Geometry check sheet. Reference: the model listing, model coordinates, mm. Face numbers are marked on the shaded views. Round coordinates to 2 decimals unless told otherwise and drop trailing zeros. Order: outer loops, then holes, each group sorted by start corner. A loop starts at its lowest first (then second) coordinate and runs counter-clockwise, first axis right, second up. Notation, with made-up numbers: M -17.75,-27.75 L -4.75,-27.75 A21 ccw -4.75,-0.75 Z; hole C 48.5,38 d10. An arc over 180 degrees is marked long. Answer as a JSON object with one key per item and string values. Group by question number.
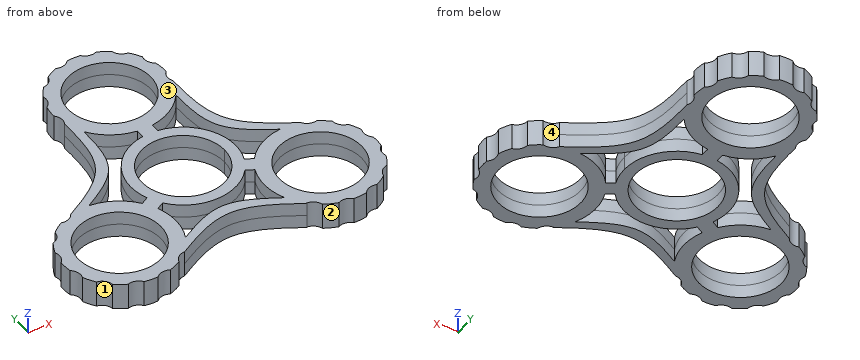
```python
from build123d import *

# Parameters (mm, degrees)
F0_R     = 11
F1_DEPTH = 3.5


with BuildPart() as f1:
    # F0 (on Top) → F1 (new body, symmetric)
    with BuildSketch(Plane.XY):
        with BuildLine():
            ThreePointArc((-12.2872806643, 22.3963534547), (-7.7936356612, 18.1836337763), (-1.9858156028, 16.1320298497))
            ThreePointArc((-1.9858156028, 16.1320298497), (0, 16), (1.9858156028, 16.1320298497))
            ThreePointArc((1.9858156028, 16.1320298497), (7.7936356612, 18.1836337763), (12.2872806643, 22.3963534547))
            ThreePointArc((12.2872806643, 22.3963534547), (13.5946168055, 24.6607260739), (14.4888873943, 27.1177143235))
            ThreePointArc((14.4888873943, 27.1177143235), (14.1339131395, 28.0975622646), (14.1302209633, 29.1397211187))
            ThreePointArc((14.1302209633, 29.1397211187), (14.4333080068, 30.0392190625), (14.9986885379, 30.8016514607))
            ThreePointArc((14.9986885379, 30.8016514607), (14.9056831484, 32.6794671415), (14.5785033995, 34.5308977089))
            ThreePointArc((14.5785033995, 34.5308977089), (13.3272676617, 36.0455189605), (13.2617309026, 38.0090294241))
            ThreePointArc((13.2617309026, 38.0090294241), (12.3374426401, 39.5315595938), (11.2392015408, 40.9337983031))
            ThreePointArc((11.2392015408, 40.9337983031), (9.4252297695, 41.6882350601), (8.449800871, 43.3935816147))
            ThreePointArc((8.449800871, 43.3935816147), (6.9211928061, 44.3077830663), (5.2949987863, 45.0343502825))
            ThreePointArc((5.2949987863, 45.0343502825), (3.3387137913, 44.8537473316), (1.6794671415, 45.9056831484))
            ThreePointArc((1.6794671415, 45.9056831484), (-0.0991764374, 45.9996721309), (-1.8764216697, 45.8821719422))
            ThreePointArc((-1.8764216697, 45.8821719422), (-3.5216132547, 44.8083874871), (-5.4801153655, 44.9631062297))
            ThreePointArc((-5.4801153655, 44.9631062297), (-7.0965596362, 44.2150989906), (-8.612945352, 43.2807643232))
            ThreePointArc((-8.612945352, 43.2807643232), (-9.5657387682, 41.562668542), (-11.3695758472, 40.7843111692))
            ThreePointArc((-11.3695758472, 40.7843111692), (-12.4491787931, 39.3676727576), (-13.3532534686, 37.8330536221))
            ThreePointArc((-13.3532534686, 37.8330536221), (-13.3928205357, 35.8688482218), (-14.6239186827, 34.3378140093))
            ThreePointArc((-14.6239186827, 34.3378140093), (-14.9164615787, 32.580877595), (-14.9986885379, 30.8016514607))
            ThreePointArc((-14.9986885379, 30.8016514607), (-14.1158588279, 29.0465787811), (-14.4888873943, 27.1177143235))
            ThreePointArc((-14.4888873943, 27.1177143235), (-13.5946168055, 24.6607260739), (-12.2872806643, 22.3963534547))
        make_face()
        with Locations((0, 31)):
            Circle(F0_R, mode=Mode.SUBTRACT)
        with BuildLine():
            Line((-1.9858156028, 16.1320298497), (-1.9858156028, 13.8584463917))
            ThreePointArc((-1.9858156028, 13.8584463917), (0, 14), (1.9858156028, 13.8584463917))
            Line((1.9858156028, 13.8584463917), (1.9858156028, 16.1320298497))
            ThreePointArc((1.9858156028, 16.1320298497), (0, 16), (-1.9858156028, 16.1320298497))
        make_face()
        with BuildLine():
            ThreePointArc((12.9946744336, -5.2094564366), (12.124355653, -7), (11.0088588308, -8.6489899551))
            Line((11.0088588308, -8.6489899551), (12.977839863, -9.7857816841))
            ThreePointArc((12.977839863, -9.7857816841), (13.8564064606, -8), (14.9636554658, -6.3462481655))
            Line((14.9636554658, -6.3462481655), (12.9946744336, -5.2094564366))
        make_face()
        with BuildLine():
            ThreePointArc((-11.0088588308, -8.6489899551), (-12.124355653, -7), (-12.9946744336, -5.2094564366))
            Line((-12.9946744336, -5.2094564366), (-14.9636554658, -6.3462481655))
            ThreePointArc((-14.9636554658, -6.3462481655), (-13.8564064606, -8), (-12.977839863, -9.7857816841))
            Line((-12.977839863, -9.7857816841), (-11.0088588308, -8.6489899551))
        make_face()
        with BuildLine():
            ThreePointArc((-1.9858156028, 13.8584463917), (-7.8443485991, 11.5959559785), (-12.124355653, 7))
            ThreePointArc((-12.124355653, 7), (-13.9645667581, 0.9954271737), (-12.9946744336, -5.2094564366))
            ThreePointArc((-12.9946744336, -5.2094564366), (-12.124355653, -7), (-11.0088588308, -8.6489899551))
            ThreePointArc((-11.0088588308, -8.6489899551), (0, -14), (11.0088588308, -8.6489899551))
            ThreePointArc((11.0088588308, -8.6489899551), (12.124355653, -7), (12.9946744336, -5.2094564366))
            ThreePointArc((12.9946744336, -5.2094564366), (13.7463711952, -2.6527870183), (14, 0))
            ThreePointArc((14, 0), (10.5783131557, 9.1705665463), (1.9858156028, 13.8584463917))
            ThreePointArc((1.9858156028, 13.8584463917), (0, 14), (-1.9858156028, 13.8584463917))
        make_face()
        with BuildLine():
            ThreePointArc((-9.5262794416, 5.5), (2.8470094961, 10.6251840892), (11, 0))
            ThreePointArc((11, 0), (-2.8470094961, -10.6251840892), (-9.5262794416, 5.5))
        make_face(mode=Mode.SUBTRACT)
        with BuildLine():
            add(Edge.make_bspline(
                [(-12.2872806643, 22.3963534547), (-12.3339502602, 17.33987948), (-12.4273981941, 7.2151497208), (-21.1653776172, 2.035672616), (-25.5394513761, -0.5570795286)],
                knots=[0, 0, 0, 0, 0.4994181667, 1, 1, 1, 1], degree=3))
            ThreePointArc((-12.2872806643, 22.3963534547), (-13.5946168055, 24.6607260739), (-14.4888873943, 27.1177143235))
            add(Edge.make_bspline(
                [(-30.7290731939, -1.0111126057), (-25.2865284697, 2.114867038), (-14.4116832718, 8.3609424382), (-14.4631688535, 20.8693847353), (-14.4888873943, 27.1177143235)],
                knots=[0, 0, 0, 0, 0.5004710067, 1, 1, 1, 1], degree=3))
            ThreePointArc((-30.7290731939, -1.0111126057), (-28.1541236585, -0.5570795286), (-25.5394513761, -0.5570795286))
        make_face()
        with BuildLine():
            ThreePointArc((14.4888873943, 27.1177143235), (13.5946168055, 24.6607260739), (12.2872806643, 22.3963534547))
            add(Edge.make_bspline(
                [(12.2872806643, 22.3963534547), (12.3023130611, 17.2868927949), (12.3323430842, 7.0797898225), (21.1404814617, 1.9865778544), (25.5394513761, -0.5570795286)],
                knots=[0, 0, 0, 0, 0.5005789276, 1, 1, 1, 1], degree=3))
            ThreePointArc((25.5394513761, -0.5570795286), (28.1541236585, -0.5570795286), (30.7290731939, -1.0111126057))
            add(Edge.make_bspline(
                [(14.4888873943, 27.1177143235), (14.4747928154, 20.8413425093), (14.446630187, 8.3004126056), (25.3050017689, 2.0907792787), (30.7290731939, -1.0111126057)],
                knots=[0, 0, 0, 0, 0.5004710067, 1, 1, 1, 1], degree=3))
        make_face()
        with BuildLine():
            ThreePointArc((14.9636554658, -6.3462481655), (13.8564064606, -8), (12.977839863, -9.7857816841))
            ThreePointArc((12.977839863, -9.7857816841), (11.8506709528, -15.8413033586), (13.2521707118, -21.8392739261))
            ThreePointArc((13.2521707118, -21.8392739261), (14.559506853, -24.1036465453), (16.2401857995, -26.1066017178))
            ThreePointArc((16.2401857995, -26.1066017178), (18.0971457035, -26.7479817318), (19.1756683745, -28.3900710276))
            ThreePointArc((19.1756683745, -28.3900710276), (20.8484071525, -29.248433838), (22.6153829316, -29.8908031476))
            ThreePointArc((22.6153829316, -29.8908031476), (24.5527012815, -29.5645118383), (26.2859196032, -30.4895105718))
            ThreePointArc((26.2859196032, -30.4895105718), (28.0666135394, -30.4503185409), (29.8301084335, -30.2003332041))
            ThreePointArc((29.8301084335, -30.2003332041), (31.3904557163, -29.0066059469), (33.3550436041, -29.0145330185))
            ThreePointArc((33.3550436041, -29.0145330185), (34.9110693177, -28.1478203278), (36.3533919945, -27.1027786032))
            ThreePointArc((36.3533919945, -27.1027786032), (37.1751277484, -25.318284625), (38.9157542138, -24.4073027836))
            ThreePointArc((38.9157542138, -24.4073027836), (39.8864728498, -22.9139467512), (40.6733373176, -21.3160571369))
            ThreePointArc((40.6733373176, -21.3160571369), (40.5660084937, -19.3543872027), (41.6792499107, -17.7356339926))
            ThreePointArc((41.6792499107, -17.7356339926), (41.8396787748, -15.9617485709), (41.7887140751, -14.1813526853))
            ThreePointArc((41.7887140751, -14.1813526853), (40.7771961905, -12.4971614918), (41.0050374719, -10.5458140707))
            ThreePointArc((41.0050374719, -10.5458140707), (40.3179940925, -8.9025312877), (39.4410122738, -7.3522700841))
            ThreePointArc((39.4410122738, -7.3522700841), (37.7597440324, -6.3359012987), (37.0493785839, -4.5042219226))
            ThreePointArc((37.0493785839, -4.5042219226), (35.6740984643, -3.3724041358), (34.1743569124, -2.4115804331))
            ThreePointArc((34.1743569124, -2.4115804331), (32.2130045314, -2.2985970493), (30.7290731939, -1.0111126057))
            ThreePointArc((30.7290731939, -1.0111126057), (28.1541236585, -0.5570795286), (25.5394513761, -0.5570795286))
            ThreePointArc((25.5394513761, -0.5570795286), (19.644306614, -2.3423304177), (14.9636554658, -6.3462481655))
        make_face()
        with Locations((26.8467875173, -15.5)):
            Circle(F0_R, mode=Mode.SUBTRACT)
        with BuildLine():
            add(Edge.make_bspline(
                [(-13.2521707118, -21.8392739261), (-8.8498138423, -19.3014829213), (-0.0348937024, -14.2200173103), (8.8197317824, -19.2975620337), (13.2521707118, -21.8392739261)],
                knots=[0, 0, 0, 0, 0.4994210724, 1, 1, 1, 1], degree=3))
            ThreePointArc((-13.2521707118, -21.8392739261), (-14.559506853, -24.1036465453), (-16.2401857995, -26.1066017178))
            add(Edge.make_bspline(
                [(16.3813667404, -26.2459279712), (10.9312657247, -23.0359426949), (0.0491808111, -16.6266427117), (-10.8164268244, -22.950124614), (-16.2401857995, -26.1066017178)],
                knots=[0, 0, 0, 0, 0.5008324286, 1, 1, 1, 1], degree=3))
            ThreePointArc((16.3813667404, -26.2459279712), (16.3105459694, -26.1764982108), (16.2401857995, -26.1066017178))
            ThreePointArc((16.2401857995, -26.1066017178), (14.559506853, -24.1036465453), (13.2521707118, -21.8392739261))
        make_face()
        with BuildLine():
            ThreePointArc((-12.977839863, -9.7857816841), (-13.8564064606, -8), (-14.9636554658, -6.3462481655))
            ThreePointArc((-14.9636554658, -6.3462481655), (-19.644306614, -2.3423304177), (-25.5394513761, -0.5570795286))
            ThreePointArc((-25.5394513761, -0.5570795286), (-28.1541236585, -0.5570795286), (-30.7290731939, -1.0111126057))
            ThreePointArc((-30.7290731939, -1.0111126057), (-32.2130045314, -2.2985970493), (-34.1743569124, -2.4115804331))
            ThreePointArc((-34.1743569124, -2.4115804331), (-35.7540903009, -3.4310333035), (-37.1938863311, -4.6400945613))
            ThreePointArc((-37.1938863311, -4.6400945613), (-37.8799689433, -6.4810071222), (-39.5476505057, -7.5195188523))
            ThreePointArc((-39.5476505057, -7.5195188523), (-40.4040561795, -9.0812410529), (-41.0693099742, -10.733465099))
            ThreePointArc((-41.0693099742, -10.733465099), (-40.8156854858, -12.6816291132), (-41.804844475, -14.3790485962))
            ThreePointArc((-41.804844475, -14.3790485962), (-41.8322621239, -16.1599627386), (-41.6483907808, -17.9315716793))
            ThreePointArc((-41.6483907808, -17.9315716793), (-40.5138415398, -19.5354627066), (-40.5952213554, -21.4983803648))
            ThreePointArc((-40.5952213554, -21.4983803648), (-39.7872964124, -23.0857253797), (-38.7969156479, -24.5661148053))
            ThreePointArc((-38.7969156479, -24.5661148053), (-37.0443952391, -25.4540002844), (-36.1991345452, -27.227472237))
            ThreePointArc((-36.1991345452, -27.227472237), (-34.7431191386, -28.2533504197), (-33.1757687231, -29.0994116379))
            ThreePointArc((-33.1757687231, -29.0994116379), (-31.2114574223, -29.0655070502), (-29.6354616248, -30.2384970985))
            ThreePointArc((-29.6354616248, -30.2384970985), (-27.8688152994, -30.4651414698), (-26.0877588052, -30.4807835381))
            ThreePointArc((-26.0877588052, -30.4807835381), (-24.3669234967, -29.5329469231), (-22.4254599012, -29.8335920868))
            ThreePointArc((-22.4254599012, -29.8335920868), (-20.7576368855, -29.2084734593), (-19.1756683745, -28.3900710276))
            ThreePointArc((-19.1756683745, -28.3900710276), (-18.0971457035, -26.7479817318), (-16.2401857995, -26.1066017178))
            ThreePointArc((-16.2401857995, -26.1066017178), (-14.559506853, -24.1036465453), (-13.2521707118, -21.8392739261))
            ThreePointArc((-13.2521707118, -21.8392739261), (-11.8506709528, -15.8413033586), (-12.977839863, -9.7857816841))
        make_face()
        with Locations((-26.8467875173, -15.5)):
            Circle(F0_R, mode=Mode.SUBTRACT)
    extrude(amount=F1_DEPTH, both=True)


solid = f1.part
```
1) Thickness scan on line 1 along Y through (x, z) = (0, -2.75); line 2 along Y through (x, z) = (23.5, -1.5); line 3 along X through (y, z) = (-23, -1.5) (3 decimals). Record the ranges inside material, lowest first. Write a range as [from, to].
2) Go/stop test with flat-tipped pins: P1, Ø2.5, axis at y = 14.5, z = 2, coming from the +X side; P2, Ø2, axis at x = -25, z = -2, coming from the -Y side; P3, Ø2.5, axis at y = 15.5, z = 2.5, coming from the -X side. Record where each tip stops, or that it passes through.
3) Sectioned sample at A-A (y = -15.5). Record the boundary of the cut face in (x, z), then the cut area to 3 significant figures.
4) Sectioned sample at B-B (y = 19). Count the separate pieces of the cut face and the enclosed holes in it, then the cut area to 3 significant figures.
5) Release check for a two-part mould opening along X. For the marked faces 1, 2, 3 and 4 record: +X half, -X half, draft (parallel to the pull), parting line (faces both ways), or undercut.
Final values:
{
 "1": {"line 1": "y = [-19.81, -16.76], [-14, -11], [11, 20], [42, 46]", "line 2": "y = [-29.58, -25.98], [-5.02, -0.88], [0.63, 3.43]", "line 3": "x = [-39.837, -34.894], [-18.8, -10.685], [10.635, 18.8], [34.894, 39.837]"},
 "2": {"P1": "stops at x = 15.73", "P2": "stops at y = -30.39", "P3": "stops at x = -15.44"},
 "3": {"outline": "M -41.85,-3.5 L -37.85,-3.5 L -37.85,3.5 L -41.85,3.5 Z; M -15.85,-3.5 L -11.85,-3.5 L -11.85,3.5 L -15.85,3.5 Z; M 11.85,-3.5 L 15.85,-3.5 L 15.85,3.5 L 11.85,3.5 Z; M 37.85,-3.5 L 41.85,-3.5 L 41.85,3.5 L 37.85,3.5 Z", "area": "112 mm^2"},
 "4": {"separate pieces": "3", "enclosed holes": "0", "area": "159 mm^2"},
 "5": {"face 1": "-X half", "face 2": "undercut", "face 3": "draft", "face 4": "undercut"}
}
